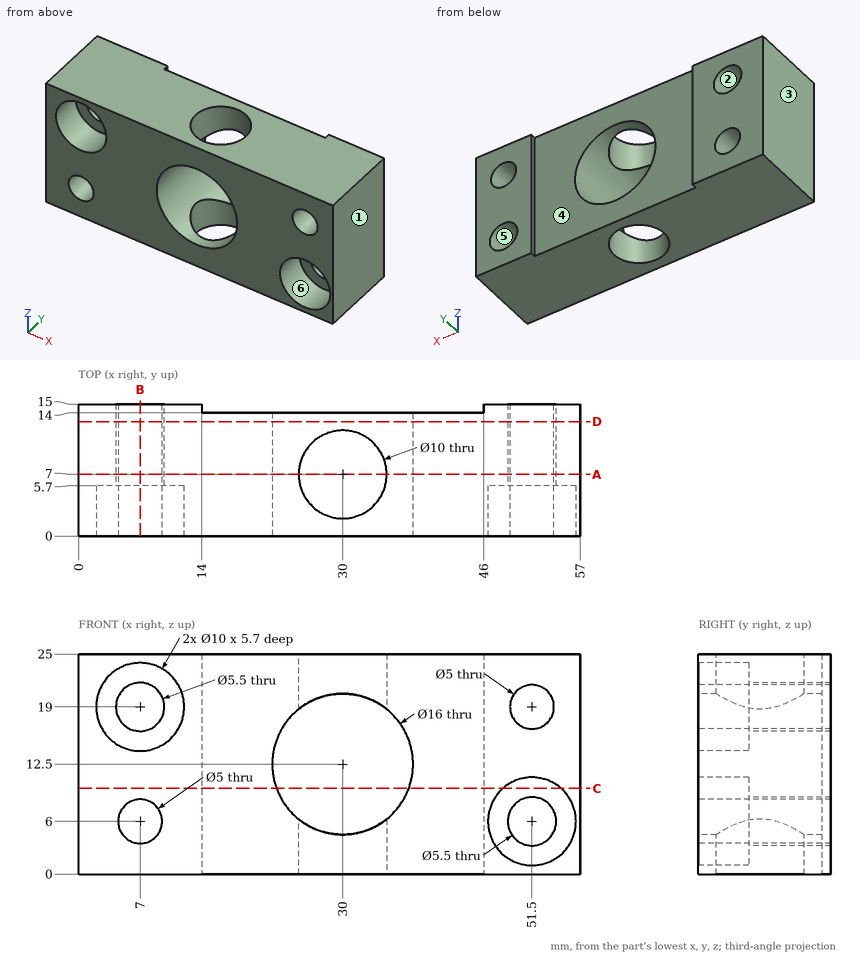
Can you work these out from the drawing? Everything is in mm from the part's minimum corner. A direction names the side the tool comes from. Coordinates: 2 decimals unless noted, no trailing zeros. Loops run counter-clockwise (first coordinate to the right, second up) from the corner with the lowest first, then second, coordinate; pieces in that order, holes last. Notation, with made-up numbers: (11, 43) - (36, 43) arc R20 ccw to (36, 61) - close; hole circle Ø2 at (3, 37). An arc over 180 degrees is marked (long way). Answer as CSV lines item,"result".
Q1. If we section it at C-C, the plane z = 9.75: Write out the boundary of the cut face in (x, y), and give its area (3 significant figures).
Response:
outline,"(0, 0) - (22.49, 0) - (22.49, 14) - (14, 14) - (14, 15) - (0, 15) - close; (37.51, 0) - (48.19, 0) - (48.19, 5.7) - (54.81, 5.7) - (54.81, 0) - (57, 0) - (57, 15) - (46, 15) - (46, 14) - (37.51, 14) - close"
area,"575 mm2"
Q2. For pin 1 (13 mm diameter, centred on x = 7, z = 19, fed in from -Y); pin 2 (4 mm diameter, centred on x = 40, z = 16, fed in from +Y); pin 3 (3 mm diameter, centred on x = 53.5, z = 4.5, fed in from -Y), each with a flat end and sliding along its axis, tell me the tip position at first contact or that it passes through.
Response:
pin 1,"y = 0"
pin 2,"y = 14"
pin 3,"y = 5.7"
Q3. If we section it at B-B, the plane x = 7: Write out the boundary of the cut face in (y, z), and give its area (3 significant figures).
Response:
outline,"(0, 0) - (15, 0) - (15, 3.5) - (0, 3.5) - close; (0, 8.5) - (15, 8.5) - (15, 16.25) - (5.7, 16.25) - (5.7, 14) - (0, 14) - close; (0, 24) - (5.7, 24) - (5.7, 21.75) - (15, 21.75) - (15, 25) - (0, 25) - close"
area,"192 mm2"
Q4. If I drill on L1, parallel to Z at x = 7, y = 3.7; L2, parallel to Z at x = 7, y = 11.75; L3, parallel to X at y = 9.5, z = 8.25, over which ranges is the centre line in solid material (lowest first)? Write a range as [from, to].
Response:
L1,"[0, 3.5], [8.5, 14], [24, 25]"
L2,"[0, 3.5], [8.5, 16.25], [21.75, 25]"
L3,"[0, 5.91], [8.09, 23.22], [36.78, 49.92], [53.08, 57]"
Q5. If we section it at A-A, the plane y = 7: Write out the boundary of the cut face in (x, z) (3 decimals), and give its area (3 significant figures).
Response:
outline,"(0, 0) - (25, 0) - (25, 6.255) arc R8 cw to (25, 18.745) - (25, 25) - (0, 25) - close; (35, 0) - (57, 0) - (57, 25) - (35, 25) - (35, 18.745) arc R8 cw to (35, 6.255) - close; hole circle Ø5.5 at (7, 19); hole circle Ø5 at (7, 6); hole circle Ø5.5 at (51.5, 6); hole circle Ø5 at (51.5, 19)"
area,"1,040 mm2"
Q6. If we section it at D-D, the plane y = 13: Write out the boundary of the cut face in (x, z).
Response:
outline,"(0, 0) - (57, 0) - (57, 25) - (0, 25) - close; hole circle Ø5.5 at (7, 19); hole circle Ø5 at (7, 6); hole circle Ø16 at (30, 12.5); hole circle Ø5.5 at (51.5, 6); hole circle Ø5 at (51.5, 19)"
Q7. For the marked faces 4, 5 and 6, which set-ups out of +Z, -Z, +X, -X, +Y, -Y let a thin tool reach every point of the face, with its end or its side?
Response:
face 4,"+Z, -Z, +Y"
face 5,"+Y, -Y"
face 6,"-Y"
Q8. We'd pull the mould along X, two halves only. Please class the marked faces 1, 2 and 3: pulls with the +X half, pulls with the -X half, needs draft (parallel to the pull), parting line crosses it, or undercut.
Response:
face 1,"pulls with the +X half"
face 2,"undercut"
face 3,"pulls with the -X half"
